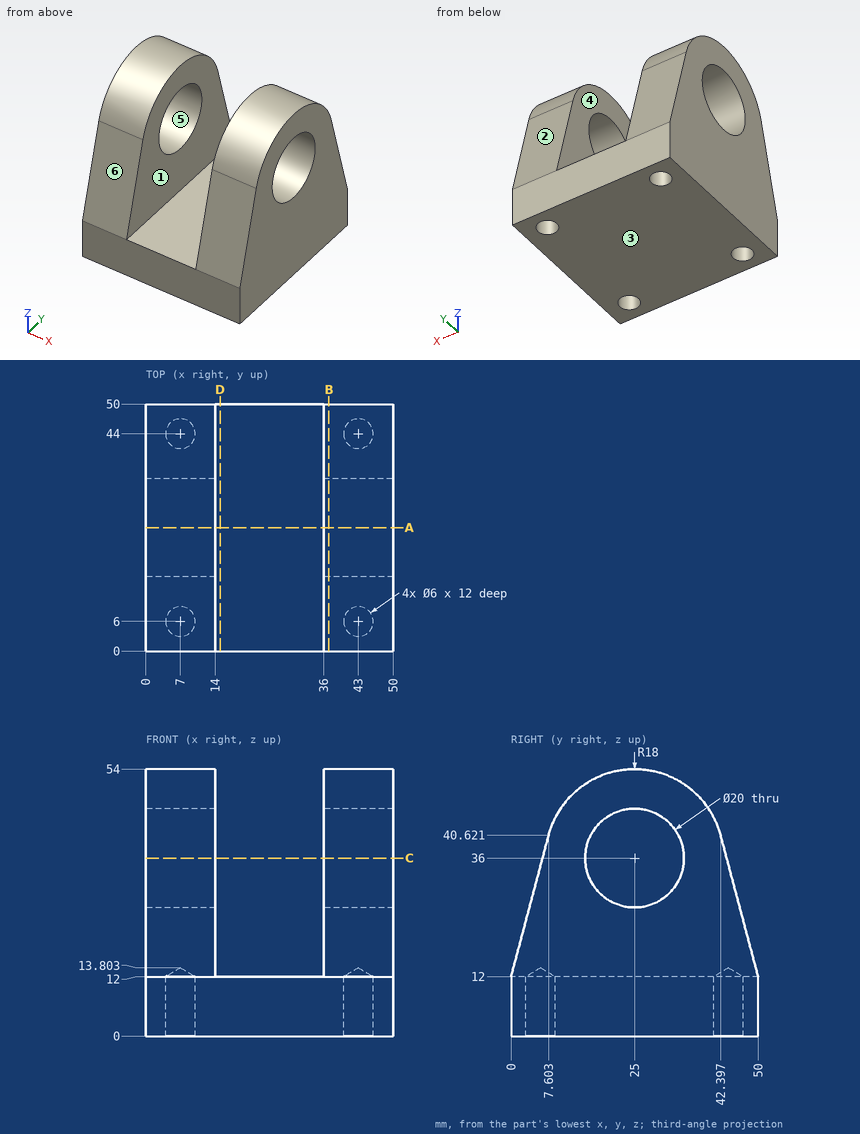
Answer from the drawing. Dimensions are ordinates in mm from the lowest x, y and z of the part. A direction names the side the tool comes from. Coordinates: 2 decimals unless noted, no trailing zeros. Loops run counter-clockwise (first coordinate to the right, second up) from the corner with the lowest first, then second, coordinate; pieces in that order, holes last. Notation, with made-up numbers: (78, -24) - (132, -24) arc R22 cw to (132, -9) - close; hole circle Ø2 at (53, -23). An arc over 180 degrees is marked (long way). Use a Markdown table: item, result.
Item 1: Find section B-B, the plane x = 37. Determine the outline of the cut face in (y, z), and give its area (3 significant figures).
Evaluation:
| item | result |
|---|---|
| outline | (0, 0) - (50, 0) - (50, 12) - (42.4, 40.62) arc R18 ccw to (7.6, 40.62) - (0, 12) - close; hole circle Ø20 at (25, 36) |
| area | 1,840 mm2 |
Item 2: Given pin 1 Ø8 at (x, z) = (42.5, 18) entering from +Y; pin 2 Ø9.5 at (x, y) = (43, 6) entering from +Z (1 decimal); pin 3 Ø6 at (x, z) = (41, 25) entering from -Y, each flat-ended and moving along its own axis, determine where each tip first touches the part or whether it passes through.
Evaluation:
| item | result |
|---|---|
| pin 1 | stops at y = 49.47 |
| pin 2 | stops at z = 47 |
| pin 3 | stops at y = 2.66 |
Item 3: For the marked faces 1 and 2, determine the directions among +Z, -Z, +X, -X, +Y, -Y from which every point of the face is accessible in a straight line to the end or side of a thin tool.
Evaluation:
| item | result |
|---|---|
| face 1 | +Z, +Y, -Y |
| face 2 | +Z, +X, -X, +Y |
Item 4: Find section A-A, the plane y = 25. Determine the outline of the cut face in (x, z).
Evaluation:
| item | result |
|---|---|
| outline | (0, 0) - (50, 0) - (50, 26) - (36, 26) - (36, 12) - (14, 12) - (14, 26) - (0, 26) - close; (0, 46) - (14, 46) - (14, 54) - (0, 54) - close; (36, 46) - (50, 46) - (50, 54) - (36, 54) - close |
Item 5: Consider probe 1 along X at (y, z) = (44, 6.25); probe 2 along X at (y, z) = (15.5, 45.5); probe 3 along Y at (x, z) = (43, 4.75). Determine where each line is inside the solid, lowest interval first. Write a range as from..to.
Evaluation:
| item | result |
|---|---|
| probe 1 | x = 0..4, 10..40, 46..50 |
| probe 2 | x = 0..14, 36..50 |
| probe 3 | y = 0..3, 9..41, 47..50 |
Item 6: The mould has two halves that part along Z. Classify the marked faces 3, 4, 5 and 6: +Z half, -Z half, draft (parallel to the pull), parting line (faces both ways), or undercut.
Evaluation:
| item | result |
|---|---|
| face 3 | -Z half |
| face 4 | draft |
| face 5 | undercut |
| face 6 | +Z half |
Item 7: Find section C-C, the plane z = 36. Determine the outline of the cut face in (x, y) (1 decimal).
Evaluation:
| item | result |
|---|---|
| outline | (0, 6.4) - (14, 6.4) - (14, 15) - (0, 15) - close; (0, 35) - (14, 35) - (14, 43.6) - (0, 43.6) - close; (36, 6.4) - (50, 6.4) - (50, 15) - (36, 15) - close; (36, 35) - (50, 35) - (50, 43.6) - (36, 43.6) - close |
Item 8: Find section D-D, the plane x = 15. Determine the outline of the cut face in (y, z).
Evaluation:
| item | result |
|---|---|
| outline | (0, 0) - (50, 0) - (50, 12) - (0, 12) - close |
